from build123d import *

# Parameters (mm, degrees)
F1_DEPTH  = 60.96
F2_W      = 1.5875
F2_H      = 32.4230269723
F3_DEPTH  = 3.175
F4_W      = 1.5875
F4_H      = 32.4230269723
F5_DEPTH  = 3.175
F7_DEPTH  = 60.961
F8_W      = 54.0470709093
F8_H      = 51.1124171317
F9_DEPTH  = 3.176
F10_W     = 1.5875
F10_H     = 25.4
F11_DEPTH = 3.175
F12_W     = 1.5875
F12_H     = 25.4
F13_DEPTH = 3.175
F15_DEPTH = 3.175
F17_DEPTH = 3.175
F18_W     = 36.9880022481
F18_H     = 16.6493579745
F19_DEPTH = 19.5074859241
F20_DEPTH = 0.396875
F21_DEPTH = 0.396875
F22_DEPTH = 19.05
F23_DEPTH = 19.05


with BuildPart() as f1:
    # F0 (on Right) → F1 (new body)
    with BuildSketch(Plane.YZ):
        Polygon((-32.4230269723, -0.8245654169), (24.7269730277, -0.8245654169), (68.72106354, 24.5754345831), (68.72106354, 27.7504345831), (24.7269730277, 2.3504345831), (-32.4230269723, 2.3504345831), align=None)
    extrude(amount=F1_DEPTH)

    # F2 (on face) → F3 (join)
    with BuildSketch(Plane.XY.offset(2.3504345831)):
        with Locations((60.16625, -16.2115134861)):
            Rectangle(F2_W, F2_H)
    extrude(amount=F3_DEPTH)

    # F4 (on face) → F5 (join)
    with BuildSketch(Plane.XY.offset(2.3504345831)):
        with Locations((0.79375, -16.2115134861)):
            Rectangle(F4_W, F4_H)
    extrude(amount=F5_DEPTH)

    # F6 (on face) → F7 (cut, through all)
    with BuildSketch(Plane.YZ.offset(60.96)):
        Polygon((68.72106354, 27.7504345831), (58.240683562, 21.6995843816), (58.240683562, 18.5245843816), (68.72106354, 24.5754345831), align=None)
    extrude(amount=-F7_DEPTH, mode=Mode.SUBTRACT)

    # F8 (on face) → F9 (cut, through all)
    with BuildSketch(Plane.XY.offset(2.3504345831)):
        with Locations((30.776332831, -3.5890638828)):
            Rectangle(F8_W, F8_H)
    extrude(amount=-F9_DEPTH, mode=Mode.SUBTRACT)

    # F10 (on face) → F11 (join)
    with BuildSketch(Plane(origin=(0, 5.1639752275, -8.944267463), x_dir=(1, 0, 0), z_dir=(0, -0.5, 0.8660254038))):
        with Locations((60.16625, 48.5877036892)):
            Rectangle(F10_W, F10_H)
    extrude(amount=F11_DEPTH)

    # F12 (on face) → F13 (join)
    with BuildSketch(Plane(origin=(0, 5.1639752275, -8.944267463), x_dir=(1, 0, 0), z_dir=(0, -0.5, 0.8660254038))):
        with Locations((0.79375, 48.5877036892)):
            Rectangle(F12_W, F12_H)
    extrude(amount=F13_DEPTH)

    # F14 (on face) → F15 (join)
    with BuildSketch(Plane.XY.offset(2.3504345831)):
        Polygon((57.7998682857, -27.7678910643), (5.1683941856, 21.967144683), (3.7527973764, 21.967144683), (3.7527973764, 20.8684690297), (56.4532540739, -29.1452724487), (57.7998682857, -29.1452724487), align=None)
    extrude(amount=-F15_DEPTH)

    # F16 (on face) → F17 (join)
    with BuildSketch(Plane.XY.offset(2.3504345831)):
        Polygon((56.3214682043, 21.967144683), (3.7527973764, -27.7384221554), (3.7527973764, -29.1452724487), (5.1683941856, -29.1452724487), (57.7998682857, 20.8684690297), (57.7998682857, 21.967144683), align=None)
    extrude(amount=-F17_DEPTH)

    # F18 (on face) → F19 (cut, through all)
    with BuildSketch(Plane(origin=(0, 5.1639752275, -8.944267463), x_dir=(1, 0, 0), z_dir=(0, -0.5, 0.8660254038))):
        with Locations((30.2279754542, 42.3330701888)):
            Rectangle(F18_W, F18_H)
    extrude(amount=-F19_DEPTH, mode=Mode.SUBTRACT)

    # F20 (add): a face of the model
    f20_faces = [f1.faces().sort_by_distance(p)[0] for p in [
        (1.5875, 46.4484109339, 16.7243997101),
    ]]
    extrude(f20_faces, amount=F20_DEPTH)

    # F21 (add): a face of the model
    f21_faces = [f1.faces().sort_by_distance(p)[0] for p in [
        (1.5875, -16.2115134861, 3.9379345831),
    ]]
    extrude(f21_faces, amount=F21_DEPTH)

    # F22 (add): a face of the model
    f22_faces = [f1.faces().sort_by_distance(p)[0] for p in [
        (0.9921875, 0, 3.9379345831),
    ]]
    extrude(f22_faces, amount=F22_DEPTH)

    # F23 (add): a face of the model
    f23_faces = [f1.faces().sort_by_distance(p)[0] for p in [
        (60.16625, 0, 3.9379345831),
    ]]
    extrude(f23_faces, amount=F23_DEPTH)


solid = f1.part
Verification items for the finished model (mm, model axes). A direction names the side the tool comes from. Coordinates: 2 decimals unless noted, no trailing zeros. Write each loop counter-clockwise with the first axis right and the second up, starting at its lowest first coordinate (ties: lowest second). Pieces come first, ordered by that corner, then holes. Notation, with made-up numbers: M 23.25,34.25 L 59.25,34.25 A24 ccw 59.25,72.25 Z; hole C 57.25,55.5 d4. An arc over 180 degrees is marked long. Use a Markdown table: item, result.
Q1. Sectioned sample at A-A, the plane x = 44. Record the boundary of the cut face in (y, z), plus the area to 3 significant figures.
Reply:
| item | result |
|---|---|
| outline | M -32.42,-0.82 L -29.15,-0.82 L -29.15,2.35 L -32.42,2.35 Z; M -17.33,-0.82 L -14.73,-0.82 L -14.73,2.35 L -17.33,2.35 Z; M 7.75,-0.82 L 10.32,-0.82 L 10.32,2.35 L 7.75,2.35 Z; M 21.97,-0.82 L 24.73,-0.82 L 35.99,5.68 L 34.62,8.06 L 24.73,2.35 L 21.97,2.35 Z; M 49.03,16.38 L 50.41,14 L 58.24,18.52 L 58.24,21.7 Z |
| area | 96.2 mm² |
Q2. Draft check along X on faces 6 (the face through (43.444, -16.799, 0.785)), 7 (the face through (3.753, -4, 1)), 8 (the face through (28.1, -1.6, -0.825)). Enter one of: +X half, -X half, draft (parallel to the pull), parting line (faces both ways), or undercut.
Reply:
| item | result |
|---|---|
| face 6 | undercut |
| face 7 | undercut |
| face 8 | draft |
Q3. Set-up check for faces 1 (the face through (1, -7, 5.525)), 2 (the face through (16.8, -15.4, 0.8)), 3 (the face through (29.969, 49.713, 15.211)), 4 (the face through (29.97, 35.29, 6.89)), 5 (the face through (1.984, 46, 17)): record each of +Z, -Z, +X, -X, +Y, -Y from which the full face is reachable in a straight line by a thin tool's end or side.
Reply:
| item | result |
|---|---|
| face 1 | +Z, +X, -X, -Y |
| face 2 | +Z, -Z |
| face 3 | -Z, -Y |
| face 4 | +Z, +Y |
| face 5 | +Z, -Y |
Q4. Sectioned sample at C-C, the plane z = 13. Record the boundary of the cut face in (x, y), plus the area to 3 significant figures.
Reply:
| item | result |
|---|---|
| outline | M 0,36.82 L 1.98,36.82 L 1.98,43.17 L 11.73,43.17 L 11.73,48.67 L 0,48.67 Z; M 48.72,43.17 L 59.37,43.17 L 59.37,36.82 L 60.96,36.82 L 60.96,48.67 L 48.72,48.67 Z |
| area | 155 mm² |
Q5. Thickness scan on line 1 (Y direction, x = 48, z = 1.25); line 2 (X direction, y = 2, z = 2); line 3 (X direction, y = 8.5, z = 2). Record the ranges inside material, lowest first.
Reply:
| item | result |
|---|---|
| line 1 | y = -32.42 to -29.15, -21.12 to -18.51, 11.56 to 14.1, 21.97 to 28.32 |
| line 2 | x = 0 to 3.75, 23.63 to 26.3, 35.2 to 37.94, 57.8 to 60.96 |
| line 3 | x = 0 to 3.75, 16.79 to 19.42, 42.08 to 44.78, 57.8 to 60.96 |
Q6. Go/stop test with flat-tipped pins: P1, Ø2, axis at y = -8, z = 8.5, coming from the -X side; P2, Ø0.5, axis at x = 60.5, y = -8.5, coming from the +Z side; P3, Ø8, axis at x = 38, z = 10.5, coming from the -Y side; P4, Ø5, axis at x = 24, y = 36, coming from the +Z side. Record where each tip stops, or that it passes through.
Reply:
| item | result |
|---|---|
| P1 | passes through |
| P2 | stops at z = 5.53 |
| P3 | stops at y = 31.91 |
| P4 | stops at z = 8.06 |
Q7. Sectioned sample at B-B, the plane y = -15.5. Record the boundary of the cut face in (x, z), plus the area to 3 significant figures.
Reply:
| item | result |
|---|---|
| outline | M 0,-0.82 L 3.75,-0.82 L 3.75,2.35 L 1.98,2.35 L 1.98,5.53 L 0,5.53 Z; M 16.7,-0.82 L 19.53,-0.82 L 19.53,2.35 L 16.7,2.35 Z; M 42.07,-0.82 L 44.82,-0.82 L 44.82,2.35 L 42.07,2.35 Z; M 57.8,-0.82 L 60.96,-0.82 L 60.96,5.53 L 59.37,5.53 L 59.37,2.35 L 57.8,2.35 Z |
| area | 51.0 mm² |
Q8. Sectioned sample at D-D, the plane x = 52. Record the boundary of the cut face in (y, z), plus the area to 3 significant figures.
Reply:
| item | result |
|---|---|
| outline | M -32.42,-0.82 L -29.15,-0.82 L -29.15,2.35 L -32.42,2.35 Z; M -24.92,-0.82 L -22.29,-0.82 L -22.29,2.35 L -24.92,2.35 Z; M 15.36,-0.82 L 17.88,-0.82 L 17.88,2.35 L 15.36,2.35 Z; M 21.97,-0.82 L 24.73,-0.82 L 58.24,18.52 L 58.24,21.7 L 24.73,2.35 L 21.97,2.35 Z |
| area | 142 mm² |
